Part model, mm, in its own coordinate system. A direction names the side the tool comes from. Round coordinates to 2 decimals unless told otherwise and drop trailing zeros. Write each loop counter-clockwise with the first axis right and the second up, starting at its lowest first coordinate (ties: lowest second). Pieces come first, ordered by that corner, then holes. Notation, with made-up numbers: M 68,80 L 85,80 A4 cw 85,85 Z; hole C 45.25,52 d4. An arc over 180 degrees is marked long. Use one line per item in the form item = value. Start each with the question number.
Item 1: Probe L1, parallel to Z at x = -20, y = 15; L2, parallel to Y at x = -23, z = 25.5; L3, parallel to Y at x = -10, z = 2.3. List the from-to ranges inside material, lowest first.
Item 2: Which spindle directions (+Z, -Z, +X, -X, +Y, -Y) get a long thin tool onto all of the face, cutting with end or side? Do faces 5 (the face through (-14.5, -3, 8)), 6 (the face through (0, -1.208, 3)), 7 (the face through (3.1, -12, 20)), 8 (the face through (-7, 16, 20)), 9 (the face through (-16.4, 16.7, 3.3)). Say none if no direction does.
Item 3: Cut at A-A, the plane x = 20. Give the cut face in (y, z) (3 decimals), then the cut area to 3 significant figures.
Item 4: Cut at C-C, the plane y = 2.5. Give the cut face in (x, z) (3 decimals), then the cut area to 3 significant figures.
Item 5: Flat gauge pins, fed straight in: pin 1 Ø7 at (x, z) = (-20, 6) entering from -Y; pin 2 Ø12 at (x, z) = (-0.5, 5.5) entering from +Y; pin 3 Ø8.5 at (x, y) = (10, -0.81) entering from +Z. Where does each tip first touch, or does it go through?
Item 6: Cut at B-B, the plane z = 21.5. Give the cut face in (x, y), then the cut area to 3 significant figures.
Item 7: Cut at D-D, the plane x = 0.5. Give the cut face in (y, z).
Item 8: Mould opens along X. For faces 1 (the face through (-17, 19.192, 20)), 2 (the face through (30.1, 3, 20)), 3 (the face through (0, 6, 11)), 4 (the face through (-24.9, 4, 25)) say: +X half, -X half, draft (parallel to the pull), parting line (faces both ways), or undercut.
from build123d import *

# Parameters (mm, degrees)
BOSS_EXTRUDE1_DEPTH = 40
SKETCH2_R           = 2.6
BOSS_EXTRUDE2_DEPTH = 11
SKETCH3_R           = 4.5
CUT_EXTRUDE1_DEPTH  = 5
CHAMFER1_SIZE       = 3
SKETCH4_R           = 2.675
CUT_EXTRUDE5_DEPTH  = 60.413887266
SKETCH5_R           = 4.5
CUT_EXTRUDE6_DEPTH  = 5
CUT_EXTRUDE7_START  = -5
CUT_EXTRUDE7_DEPTH  = 5


# Read off the part's stored shape, not the designer's step: Cut-Extrude7
with BuildPart() as part:
    # Sketch1 → Boss-Extrude1 (new body)
    with BuildSketch(Plane.XY):
        Polygon((-29.9, 19.191927939), (-29.9, -10.808072061), (-2.9, -10.808072061), (-2.9, -12.808072061), (3.1, -12.808072061), (3.1, -10.808072061), (30.1, -10.808072061), (30.1, 19.191927939), (7, 19.191927939), (7, 13.191927939), (24.9, 13.191927939), (24.9, -5.808072061), (5.6, -5.808072061), (-5.4, -5.808072061), (-24.9, -5.808072061), (-24.9, 13.191927939), (-7, 13.191927939), (-7, 19.191927939), align=None)
    extrude(amount=BOSS_EXTRUDE1_DEPTH)

    # Sketch2 → Boss-Extrude2 (add)
    with BuildSketch(Plane(origin=(0, 0, 0), x_dir=(-1, 0, 0), z_dir=(0, 0, -1))):
        Polygon((-7, 10.191927939), (-7, 13.191927939), (-24.9, 13.191927939), (-24.9, -5.808072061), (-5.6, -5.808072061), (-5.6, -2.208368155), (-4.6, -1.208368155), (4.4, -1.208368155), (5.4, -2.208368155), (5.4, -5.808072061), (24.9, -5.808072061), (24.9, 13.191927939), (7, 13.191927939), (7, 10.191927939), align=None)
        with Locations((-10, -0.808072061)):
            Circle(SKETCH2_R, mode=Mode.SUBTRACT)
        with Locations((10, -0.808092061)):
            Circle(SKETCH2_R, mode=Mode.SUBTRACT)
    extrude(amount=-BOSS_EXTRUDE2_DEPTH)

    # Sketch3 → Cut-Extrude1 (cut)
    with BuildSketch(Plane.XY.offset(11)):
        with Locations((-10, -0.808092061)):
            Circle(SKETCH3_R)
        with Locations((10, -0.808072061)):
            Circle(SKETCH3_R)
    extrude(amount=-CUT_EXTRUDE1_DEPTH, mode=Mode.SUBTRACT)

    # Chamfer1
    chamfer1_edges = [part.edges().sort_by_distance(p)[0] for p in [
        (-29.9, 19.191927939, 20),
        (30.1, 19.191927939, 20),
    ]]
    chamfer(chamfer1_edges, length=CHAMFER1_SIZE)

    # Sketch4 → Cut-Extrude5 (cut, through all)
    with BuildSketch(Plane(origin=(0, 19.191927939, 0), x_dir=(1, 0, 0), z_dir=(0, 1, 0))):
        with Locations(Location((-20, -6, 0), (0, 0, 180))):
            Circle(SKETCH4_R)
        with Locations(Location((20, -6, 0), (0, 0, 270))):
            Circle(SKETCH4_R)
    extrude(amount=-CUT_EXTRUDE5_DEPTH, mode=Mode.SUBTRACT)

    # Sketch5 → Cut-Extrude6 (cut)
    with BuildSketch(Plane(origin=(0, 19.191927939, 0), x_dir=(1, 0, 0), z_dir=(0, 1, 0))):
        with Locations(Location((-20, -6, 0), (0, 0, 180))):
            Circle(SKETCH5_R)
        with Locations((20, -6)):
            Circle(SKETCH5_R)
    extrude(amount=-CUT_EXTRUDE6_DEPTH, mode=Mode.SUBTRACT)

    # Cut-Extrude7 outline → Cut-Extrude7 (cut)
    with BuildSketch(Plane.XY.offset(11).offset(CUT_EXTRUDE7_START)):
        with BuildLine():
            Line((9.9999955, 3.691927939), (-10.0000045, 3.691907939))
            ThreePointArc((-10.0000045, 3.691907939), (-6.818017894, -3.990070985), (-14.5, -0.808092061))
            Line((-14.5, -0.808092061), (-14.5, -5.808072061))
            Line((-14.5, -5.808072061), (-5.4, -5.808072061))
            Line((-5.4, -5.808072061), (-5.4, -2.208368155))
            Line((-5.4, -2.208368155), (-4.4, -1.208368155))
            Line((-4.4, -1.208368155), (4.6, -1.208368155))
            Line((4.6, -1.208368155), (5.6, -2.208368155))
            Line((5.6, -2.208368155), (5.6, -5.808072061))
            Line((5.6, -5.808072061), (14.5, -5.808072061))
            Line((14.5, -5.808072061), (14.5, -0.808072061))
            ThreePointArc((14.5, -0.808072061), (6.818021076, -3.990054167), (9.9999955, 3.691927939))
        make_face()
    extrude(amount=CUT_EXTRUDE7_DEPTH, mode=Mode.SUBTRACT)


solid = part.part
Model answer:
q1.L1 = 0 to 1.5, 10.5 to 40
q1.L2 = -10.81 to -5.81, 13.19 to 19.19
q1.L3 = -10.81 to -3.41, 1.79 to 19.19
q2.face_5 = +Z
q2.face_6 = +Z, -Z
q2.face_7 = +Z, -Z, +X, -Y
q2.face_8 = +Z, -Z, +Y
q2.face_9 = +Y
q3.outline = M -10.808,0 L 19.192,0 L 19.192,1.5 L 14.192,1.5 L 14.192,3.325 L -10.808,3.325 Z; M -10.808,8.675 L 14.192,8.675 L 14.192,10.5 L 19.192,10.5 L 19.192,40 L 13.192,40 L 13.192,11 L -5.808,11 L -5.808,40 L -10.808,40 Z
q3.area = 470 mm²
q4.outline = M -29.9,0 L 30.1,0 L 30.1,40 L 24.9,40 L 24.9,11 L 13.051,11 L 13.051,6 L -13.051,6 L -13.051,11 L -24.9,11 L -24.9,40 L -29.9,40 Z; hole C -20,6 d5.35; hole C 20,6 d5.35
q4.area = 780 mm²
q5.pin_1 = -10.81
q5.pin_2 = 10.19
q5.pin_3 = 6
q6.outline = M -29.9,-10.81 L -2.9,-10.81 L -2.9,-12.81 L 3.1,-12.81 L 3.1,-10.81 L 30.1,-10.81 L 30.1,16.19 L 27.1,19.19 L 7,19.19 L 7,13.19 L 24.9,13.19 L 24.9,-5.81 L -24.9,-5.81 L -24.9,13.19 L -7,13.19 L -7,19.19 L -26.9,19.19 L -29.9,16.19 Z
q6.area = 773 mm²
q7.outline = M -12.81,0 L -5.81,0 L -5.81,40 L -12.81,40 Z; M -1.21,0 L 10.19,0 L 10.19,11 L 3.69,11 L 3.69,6 L -1.21,6 Z
q8.face_1 = draft
q8.face_2 = +X half
q8.face_3 = undercut
q8.face_4 = undercut
